from build123d import *

# Parameters (mm, degrees)
SKETCH1_W                       = 46
SKETCH1_H                       = 32
BOSS_EXTRUDE1_DEPTH             = 20.6
M2X0_4_TAPPED_HOLE1_D           = 1.6
M2X0_4_TAPPED_HOLE1_DEPTH       = 6
M2X0_4_TAPPED_HOLE1_CSINK_D     = 2.05
M2X0_4_TAPPED_HOLE1_CSINK_ANGLE = 90
M2X0_4_TAPPED_HOLE1_TIP         = 0.480688495
FILLET1_R                       = 1.6
SKETCH4_R                       = 6
BOSS_EXTRUDE2_DEPTH             = 0.5
CUT_EXTRUDE3_DEPTH              = 18.8
SKETCH6_W                       = 2
SKETCH6_H                       = 22
CUT_EXTRUDE1_DEPTH              = 17.8
SKETCH7_W                       = 1
SKETCH7_H                       = 22.4
CUT_EXTRUDE2_DEPTH              = 17.8
SKETCH9_R                       = 3
CUT_EXTRUDE4_DEPTH              = 54.077396319
CHAMFER1_SIZE                   = 4.5
CHAMFER1_SIZE_2                 = 1.205771366


with BuildPart() as part:
    # Sketch1 → Boss-Extrude1 (new body)
    with BuildSketch(Plane(origin=(0, 0, 0), x_dir=(1, 0, 0), z_dir=(0, 1, 0))):
        with Locations((9, 0)):
            Rectangle(SKETCH1_W, SKETCH1_H)
    extrude(amount=-BOSS_EXTRUDE1_DEPTH)

    # M2x0.4 Tapped Hole1
    with Locations(Plane(origin=(0, 0, 0), x_dir=(1, 0, 0), z_dir=(0, 1, 0))):
        with Locations((-12.4, 14.4), (20.6, 14.4), (30.4, -14.4), (-12.4, -14.4)):
            CounterSinkHole(M2X0_4_TAPPED_HOLE1_D / 2, M2X0_4_TAPPED_HOLE1_CSINK_D / 2, depth=M2X0_4_TAPPED_HOLE1_DEPTH, counter_sink_angle=M2X0_4_TAPPED_HOLE1_CSINK_ANGLE)
            with Locations((0, 0, -(M2X0_4_TAPPED_HOLE1_DEPTH + M2X0_4_TAPPED_HOLE1_TIP / 2))):  # 118° drill point
                Cone(0, M2X0_4_TAPPED_HOLE1_D / 2, M2X0_4_TAPPED_HOLE1_TIP, mode=Mode.SUBTRACT)

    # Fillet1
    fillet1_edges = [part.edges().sort_by_distance(p)[0] for p in [
        (-14, -10.3, -16),
        (32, -10.3, -16),
        (32, -10.3, 16),
        (-14, -10.3, 16),
    ]]
    fillet(fillet1_edges, radius=FILLET1_R)

    # Sketch4 → Boss-Extrude2 (add)
    with BuildSketch(Plane(origin=(0, -20.6, 0), x_dir=(-1, 0, 0), z_dir=(0, -1, 0))):
        with Locations(Location((0, 0, 0), (0, 0, 270))):
            Circle(SKETCH4_R)
    extrude(amount=BOSS_EXTRUDE2_DEPTH)

    # Sketch8 → Cut-Extrude3 (cut)
    with BuildSketch(Plane(origin=(0, 0, 0), x_dir=(1, 0, 0), z_dir=(0, 1, 0))):
        with BuildLine():
            Line((-10.4, 14.4), (18.6, 14.4))
            ThreePointArc((18.6, 14.4), (20.6, 12.4), (22.6, 14.4))
            Line((22.6, 14.4), (30.4, 14.4))
            Line((30.4, 14.4), (30.4, -12.4))
            ThreePointArc((30.4, -12.4), (28.985786438, -12.985786438), (28.4, -14.4))
            Line((28.4, -14.4), (-10.4, -14.4))
            ThreePointArc((-10.4, -14.4), (-10.985786438, -12.985786438), (-12.4, -12.4))
            Line((-12.4, -12.4), (-12.4, 12.4))
            ThreePointArc((-12.4, 12.4), (-10.985786438, 12.985786438), (-10.4, 14.4))
        make_face()
    extrude(amount=-CUT_EXTRUDE3_DEPTH, mode=Mode.SUBTRACT)

    # Sketch6 → Cut-Extrude1 (cut)
    with BuildSketch(Plane(origin=(0, 0, 0), x_dir=(1, 0, 0), z_dir=(0, 1, 0))):
        with Locations((-13, 0)):
            Rectangle(SKETCH6_W, SKETCH6_H)
    extrude(amount=-CUT_EXTRUDE1_DEPTH, mode=Mode.SUBTRACT)

    # Sketch7 → Cut-Extrude2 (cut)
    with BuildSketch(Plane(origin=(0, 0, 0), x_dir=(1, 0, 0), z_dir=(0, 1, 0))):
        with Locations((-13.5, 0)):
            Rectangle(SKETCH7_W, SKETCH7_H)
    extrude(amount=-CUT_EXTRUDE2_DEPTH, mode=Mode.SUBTRACT)

    # Sketch9 → Cut-Extrude4 (cut, through all)
    with BuildSketch(Plane(origin=(32, 0, 0), x_dir=(0, 0, -1), z_dir=(1, 0, 0))):
        with Locations((2.5, -11.2)):
            Circle(SKETCH9_R)
    extrude(amount=-CUT_EXTRUDE4_DEPTH, mode=Mode.SUBTRACT)

    # Chamfer1
    # the kernel refuses this chamfer: 4.5, 1.205771366 mm, written as the material it takes off along each edge
    with BuildSketch(Plane(origin=(42.085247066, -20.6, 16), x_dir=(0, -0.009967146577156305, -0.9999503267608394), z_dir=(-1, 0, 0))) as chamfer1_piece_1:
        Polygon((CHAMFER1_SIZE * 0.999950326761, -CHAMFER1_SIZE * 0.00996714657716), (-CHAMFER1_SIZE_2 * 0.00996714657666, -CHAMFER1_SIZE_2 * 0.999950326711), (0, 0), align=None)
    extrude(amount=66.170494132, mode=Mode.SUBTRACT)
    with BuildSketch(Plane(origin=(-14, -20.6, 26.085247066), x_dir=(0.9999503267608394, -0.009967146577156305, 0), z_dir=(0, 0, -1)), Plane(origin=(32, -20.6, -26.085247066), x_dir=(-0.9999503267608394, -0.009967146577156302, 0), z_dir=(0, 0, 1))) as chamfer1_piece_2:
        Polygon((CHAMFER1_SIZE * 0.999950326761, -CHAMFER1_SIZE * 0.00996714657716), (-CHAMFER1_SIZE_2 * 0.00996714657666, -CHAMFER1_SIZE_2 * 0.999950326711), (0, 0), align=None)
    extrude(amount=52.170494132, mode=Mode.SUBTRACT)
    with BuildSketch(Plane(origin=(-24.085247066, -20.6, -16), x_dir=(0, 0.9905000388259543, -0.1375124470212905), z_dir=(1, 0, 0))) as chamfer1_piece_3:
        Polygon((CHAMFER1_SIZE_2 * 0.990500038777, CHAMFER1_SIZE_2 * 0.137512447014), (-CHAMFER1_SIZE * 0.137512447021, CHAMFER1_SIZE * 0.990500038826), (0, 0), align=None)
    extrude(amount=66.170494132, mode=Mode.SUBTRACT)


solid = part.part
Geometry check sheet. Reference: the model listing, model coordinates, mm. A direction names the side the tool comes from. Round coordinates to 2 decimals unless told otherwise and drop trailing zeros. Loops run counter-clockwise (first coordinate to the right, second up) from the corner with the lowest first, then second, coordinate; pieces in that order, holes last.
Item 1: Access from +Z, -Z, +X, -X, +Y, -Y to the whole of each face (thin tool, end or side, straight path). Record for faces 4 (the flat face through (-13.5, -8.8, 11.2)), 5 (the cylindrical face through (-11.77, -3.15, 14.89)), 6 (the flat face through (9, -10, 16)).
Item 2: Cross-section at B-B on x = 17. Record the boundary of the cut face in (y, z), then the cut area to 3 significant figures.
Item 3: Thickness scan on line 1 (Z direction, x = 2, y = -9); line 2 (Z direction, x = -12, y = -1); line 3 (X direction, y = -18.75, z = -10). Record the ranges inside material, lowest first.
Item 4: Cross-section at D-D on y = -7. Record the boundary of the cut face in (x, z), then the cut area to 3 significant figures.
Item 5: Gauge pin test, flat ends, axial feed: pin 1 (1.1 mm diameter, centred on x = -13.5, y = -10.5, fed in from +Z); pin 2 (1.8 mm diameter, centred on x = -12.4, z = -14.4, fed in from -Y); pin 3 (6 mm diameter, centred on x = 17.5, z = -4, fed in from -Y). Record the tip position at first contact, or that the pin passes through.
Item 6: Mould release check, pull along X, two halves, no side actions. Record for faces 1 (the flat face through (-14, -18, 0)), 2 (the cylindrical face through (31.52, -9.9, -15.54)), 3 (the conical face through (30.29, -6.4, 14.48)): pulls with the +X half, pulls with the -X half, needs draft (parallel to the pull), parting line crosses it, or undercut.
Item 7: Cross-section at C-C on z = 0. Record the boundary of the cut face in (x, y).
Answer sheet:
1. face 4: -X, +Y
1. face 5: +Y
1. face 6: +Z, +X, -X, +Y, -Y
2. outline: (-20.6, -11.5) - (-19.39, -16) - (0, -16) - (0, -14.4) - (-18.8, -14.4) - (-18.8, 14.4) - (0, 14.4) - (0, 16) - (-19.39, 16) - (-20.6, 11.5) - close
2. area: 112 mm2
3. line 1: z = -16 to -14.4, 14.4 to 16
3. line 2: z = -16 to -15.09, -13.71 to -12.44, 12.44 to 13.71, 15.09 to 16
3. line 3: x = -14 to -12.4, 30.4 to 32
4. outline: (-14, -14.4) arc R1.6 ccw to (-12.4, -16) - (30.4, -16) arc R1.6 ccw to (32, -14.4) - (32, 14.4) arc R1.6 ccw to (30.4, 16) - (-12.4, 16) arc R1.6 ccw to (-14, 14.4) - (-14, 11.2) - (-13, 11.2) - (-13, 11) - (-12.4, 11) - (-12.4, 12.4) arc R2 ccw to (-10.4, 14.4) - (28.4, 14.4) arc R2 ccw to (30.4, 12.4) - (30.4, -14.4) - (22.6, -14.4) arc R2 ccw to (18.6, -14.4) - (-10.4, -14.4) arc R2 ccw to (-12.4, -12.4) - (-12.4, -11) - (-13, -11) - (-13, -11.2) - (-14, -11.2) - close
4. area: 217 mm2
5. pin 1: stops at z = 15.9
5. pin 2: stops at y = -19.99
5. pin 3: stops at y = -20.6
6. face 1: pulls with the -X half
6. face 2: pulls with the +X half
6. face 3: undercut
7. outline: (-14, -19.39) - (-9.5, -20.6) - (-6, -20.6) - (-6, -21.1) - (6, -21.1) - (6, -20.6) - (27.5, -20.6) - (32, -19.39) - (32, -12.86) - (30.4, -12.86) - (30.4, -18.8) - (-12.4, -18.8) - (-12.4, -17.8) - (-14, -17.8) - close; (30.4, -9.54) - (32, -9.54) - (32, 0) - (30.4, 0) - close
